```python
from build123d import *

# Parameters (mm, degrees)
EXTRUDE_1_DEPTH     = 4
SKETCH_2_W          = 6.166461301
SKETCH_2_H          = 14.966809979
CUT_EXTRUDE_1_DEPTH = 86.646256186
CHAMFER_3_SIZE      = 1.5


with BuildPart() as part:
    # Эскиз1 → Бобышка-Вытянуть1 (new body)
    with BuildSketch(Plane.XY):
        with BuildLine():
            Line((0, 0), (0, 85.257675306))
            Line((0, 85.257675306), (-1.1, 85.257675306))
            ThreePointArc((-1.1, 85.257675306), (-5.342640687, 83.500315993), (-7.1, 79.257675306))
            Line((-7.1, 79.257675306), (-7.1, 45.60252186))
            ThreePointArc((-7.1, 45.60252186), (-6.504790591, 37.910534687), (-4.733333333, 30.40168124))
            ThreePointArc((-4.733333333, 30.40168124), (-1.190418818, 15.383974346), (0, 0))
        make_face()
    extrude(amount=EXTRUDE_1_DEPTH)

    # Эскиз2 → Вырез-Вытянуть1 (cut, through all)
    with BuildSketch(Plane.XY.offset(4)):
        with Locations((-0.950413373, 6.187246753)):
            Rectangle(SKETCH_2_W, SKETCH_2_H)
    extrude(amount=-CUT_EXTRUDE_1_DEPTH, mode=Mode.SUBTRACT)

    # Фаска3
    chamfer_3_edges = [part.edges().sort_by_distance(p)[0] for p in [
        (0, 49.464163524, 4),
    ]]
    chamfer(chamfer_3_edges, length=CHAMFER_3_SIZE)

    # Фаска4
    # the kernel refuses this chamfer: 1.5 mm, written as the material it takes off along each edge
    with BuildSketch(Plane(origin=(-100, 0, 4), x_dir=(0.9526666666666831, 0.30401681240054956, 0), z_dir=(-0.30401681240054956, 0.9526666666666831, 0))) as chamfer_4_piece_1:
        with BuildLine():
            Line((99.681801948, 1.818198052), (101.818198052, -0.318198052))
            Line((101.818198052, -0.318198052), (101.818198052, -0.543198052))
            ThreePointArc((101.818198052, -0.543198052), (100.909099026, -0.225), (100, -0.225))
            Line((100, -0.225), (99.775, 0))
            ThreePointArc((99.775, 0), (99.775, 0.909099026), (99.456801948, 1.818198052))
            Line((99.456801948, 1.818198052), (99.681801948, 1.818198052))
        make_face()
    revolve(axis=Axis((-100, 0, 4), (0, 0, -1)), revolution_arc=10.406622552, mode=Mode.SUBTRACT)
    with BuildSketch(Plane(origin=(-1.1, 79.257675306, 4), x_dir=(0.6462526290472239, 0.7631235414069935, 0), z_dir=(0.7631235414069935, -0.6462526290472239, 0))) as chamfer_4_piece_2:
        with BuildLine():
            Line((6.318198052, -1.818198052), (4.181801948, 0.318198052))
            Line((4.181801948, 0.318198052), (4.181801948, 0.543198052))
            ThreePointArc((4.181801948, 0.543198052), (5.090900974, 0.225), (6, 0.225))
            Line((6, 0.225), (6.225, 0))
            ThreePointArc((6.225, 0), (6.225, -0.909099026), (6.543198052, -1.818198052))
            Line((6.543198052, -1.818198052), (6.318198052, -1.818198052))
        make_face()
    revolve(axis=Axis((-1.1, 79.257675306, 4), (0, 0, 1)), revolution_arc=130.259658386, mode=Mode.SUBTRACT)
    with BuildSketch(Plane(origin=(42.9, 45.60252186, 4), x_dir=(-1, 0, 0), z_dir=(0, 1, 0))) as chamfer_4_piece_3:
        with BuildLine():
            Line((48.181801948, 0.318198052), (50.318198052, -1.818198052))
            Line((50.318198052, -1.818198052), (50.543198052, -1.818198052))
            ThreePointArc((50.543198052, -1.818198052), (50.225, -0.909099026), (50.225, 0))
            Line((50.225, 0), (50, 0.225))
            ThreePointArc((50, 0.225), (49.090900974, 0.225), (48.181801948, 0.543198052))
            Line((48.181801948, 0.543198052), (48.181801948, 0.318198052))
        make_face()
    revolve(axis=Axis((42.9, 45.60252186, 4), (0, 0, 1)), revolution_arc=17.69902277, mode=Mode.SUBTRACT)
    with BuildSketch(Plane(origin=(-7.1, 79.257675306, 4), x_dir=(0.9850292351397438, 0, 0.17238737169529317), z_dir=(0, -1, 0))) as chamfer_4_piece_4:
        with BuildLine():
            Line((1.845831562, 0), (-0.626868767, -1.73612491))
            Line((-0.626868767, -1.73612491), (-0.848500345, -1.697337752))
            ThreePointArc((-0.848500345, -1.697337752), (-0.37834877, -0.856701959), (-0.221631578, 0.038787159))
            Line((-0.221631578, 0.038787159), (0.038787159, 0.221631578))
            ThreePointArc((0.038787159, 0.221631578), (0.934276277, 0.064914386), (1.88461872, 0.221631578))
            Line((1.88461872, 0.221631578), (1.845831562, 0))
        make_face()
    extrude(amount=33.655153446, mode=Mode.SUBTRACT)


solid = part.part
```
Could you check a few things on this model? Use its own coordinates, in mm. Give positions to 0.01 mm unless a question says otherwise; leave off trailing zeros. Write each loop counter-clockwise with the first axis right and the second up, starting at its lowest first coordinate (ties: lowest second). Pieces come first, ordered by that corner, then holes. Notation, with made-up numbers: (48, 75.25) - (64, 75.25) arc R30 cw to (64, 104.25) - close; hole circle Ø5 at (84.5, 76.5). An arc over 180 degrees is marked (long way). One line per item, written item: value. Start each with the question number.
Item 1: Imagine slicing it at B-B, the plane y = 63.5. List the corners of the cut face in (x, z) for me, and give its area (4 significant figures).
Item 2: Imagine slicing it at A-A, the plane z = 0.75. List the corners of the cut face in (x, y) for me.
Item 3: I'm going to push flat-ended pins straight in: pin 1 (1.5 mm diameter, centred on y = 62.5, z = 3.5, fed in from -X); pin 2 (1 mm diameter, centred on x = -4.5, z = 1, fed in from +Y). Where does each tip first touch, or does it pass through?
Item 4: Please list where these lines run through material, in increasing order: line 1 (X direction, y = 33.5, z = 0.3); line 2 (Z direction, x = -6.25, y = 52.5); line 3 (Z direction, x = -3.5, y = 30). Write a range as from..to.
Geometry says:
1. outline: (-7.1, 0) - (0, 0) - (0, 2.5) - (-1.5, 4) - (-5.6, 4) - (-7.1, 2.5) - close
1. area: 26.15 mm^2
2. outline: (-7.1, 45.6) arc R50 ccw to (-4.73, 30.4) arc R100 cw to (-0.94, 13.67) - (0, 13.67) - (0, 85.26) - (-1.1, 85.26) arc R6 ccw to (-7.1, 79.26) - close
3. pin 1: x = -6.85
3. pin 2: y = 84.51
4. line 1: -5.61..0
4. line 2: 0..3.35
4. line 3: 0..3.56
